Check sheet for the modelled part. Datum: model origin and axes. Units: mm. A direction names the side the tool comes from. Coordinates: 2 decimals unless noted, no trailing zeros. Write each loop counter-clockwise with the first axis right and the second up, starting at its lowest first coordinate (ties: lowest second). Pieces come first, ordered by that corner, then holes. Notation, with made-up numbers: (-27.5, 76) - (-2.5, 76) arc R28 ccw to (-2.5, 109) - close; hole circle Ø4 at (5, 12). An arc over 180 degrees is marked (long way). Use one line per item in the form item = value. Start each with the question number.
1. Cross-section at D-D on z = 1.75. Record the boundary of the cut face in (x, y).
2. Go/stop test with flat-tipped pins: pin 1 Ø4 at (x, y) = (-0.5, 2.5) entering from -Z; pin 2 Ø4.5 at (x, z) = (0, 5) entering from +Y; pin 3 Ø4 at (x, y) = (1, -3.5) entering from -Z. Record where each tip stops, or that it passes through.
3. Draft check along X on faces 3 (the face through (-5, -4, 7)), 4 (the face through (-0.37, -4.26, 3.34)), 5 (the face through (-1, -3.5, 3)). Enter one of: +X half, -X half, draft (parallel to the pull), parting line (faces both ways), or undercut.
4. Cross-section at A-A on y = 0. Record the boundary of the cut face in (x, z), then the cut area to 4 significant figures.
5. Cross-section at C-C on z = 8.75. Record the boundary of the cut face in (x, y), then the cut area to 3 significant figures.
6. Cross-section at B-B on x = -1.5. Record the boundary of the cut face in (y, z), then the cut area to 4 significant figures.
7. Tool access check on faces 1 (the face through (0, -5, 3)), 2 (the face through (-2, 1, 8.5)). Record the directions out of +Z, -Z, +X, -X, +Y, -Y that give a thin tool (end or side, any length) a straight path to the whole face; none if there is none.
8. Scan lines: line 1 along Z through (x, y) = (4.7, 0); line 2 along Y through (x, z) = (0, 9.5); line 3 along Y through (x, z) = (-2.5, 5.75). Record each from-to range of solid material in increasing order.
```python
from build123d import *

# Parameters (mm, degrees)
F0_W     = 10
F0_H     = 10
F1_DEPTH = 10
F2_W     = 8.5
F2_H     = 8.5
F3_DEPTH = 8.5
F4_R     = 1.7
F5_DEPTH = 25
F6_R     = 1.7
F7_DEPTH = 25
F8_R     = 1.7
F9_DEPTH = 25


with BuildPart() as f1:
    # F0 (on Top) → F1 (new body)
    with BuildSketch(Plane.XY):
        Rectangle(F0_W, F0_H)
    extrude(amount=F1_DEPTH)

    # F2 (on face) → F3 (cut)
    with BuildSketch(Plane(origin=(0, 0, 0), x_dir=(1, 0, 0), z_dir=(0, 0, -1))):
        with Locations((-0.75, -0.75)):
            Rectangle(F2_W, F2_H)
    extrude(amount=-F3_DEPTH, mode=Mode.SUBTRACT)

    # F4 (on face) → F5 (cut)
    with BuildSketch(Plane.YZ.offset(5)):
        with Locations((0, 5)):
            Circle(F4_R)
    extrude(amount=-F5_DEPTH, mode=Mode.SUBTRACT)

    # F6 (on face) → F7 (cut)
    with BuildSketch(Plane.XY.offset(10)):
        Circle(F6_R)
    extrude(amount=-F7_DEPTH, mode=Mode.SUBTRACT)

    # F8 (on face) → F9 (cut)
    with BuildSketch(Plane.XZ.offset(5)):
        with Locations((0, 5)):
            Circle(F8_R)
    extrude(amount=-F9_DEPTH, mode=Mode.SUBTRACT)


solid = f1.part
```
Final values:
q1.outline = (-5, -5) - (5, -5) - (5, 5) - (3.5, 5) - (3.5, -3.5) - (-5, -3.5) - close
q2.pin_1 = 8.5
q2.pin_2 = -3.5
q2.pin_3 = 0
q3.face_3 = -X half
q3.face_4 = undercut
q3.face_5 = draft
q4.outline = (-5, 8.5) - (-1.7, 8.5) - (-1.7, 10) - (-5, 10) - close; (1.7, 8.5) - (3.5, 8.5) - (3.5, 6.7) - (5, 6.7) - (5, 10) - (1.7, 10) - close; (3.5, 0) - (5, 0) - (5, 3.3) - (3.5, 3.3) - close
q4.area = 17.55 mm²
q5.outline = (-5, -5) - (5, -5) - (5, 5) - (-5, 5) - close; hole circle Ø3.4 at (0, 0)
q5.area = 90.9 mm²
q6.outline = (-5, 0) - (-3.5, 0) - (-3.5, 4.2) - (-5, 4.2) - close; (-5, 5.8) - (-3.5, 5.8) - (-3.5, 8.5) - (-0.8, 8.5) - (-0.8, 10) - (-5, 10) - close; (0.8, 8.5) - (5, 8.5) - (5, 10) - (0.8, 10) - close
q6.area = 22.95 mm²
q7.face_1 = +Z, -Z, +X, -X, -Y
q7.face_2 = -Z, -X, +Y
q8.line_1 = 0 to 3.3, 6.7 to 10
q8.line_2 = -5 to -1.7, 1.7 to 5
q8.line_3 = -5 to -3.5
